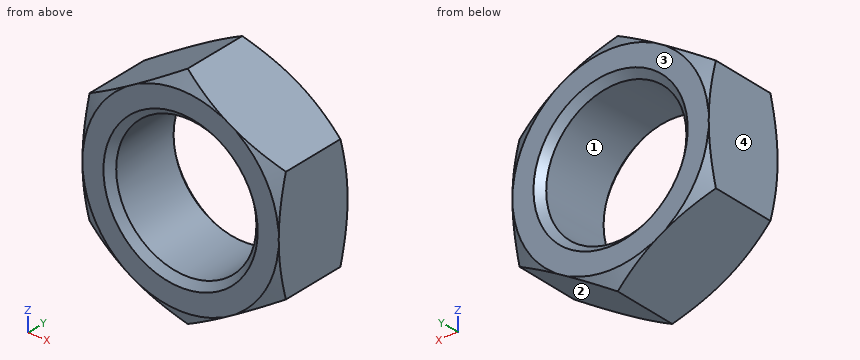
```python
from build123d import *

# Parameters (mm, degrees)
BOSS_EXTRUDE1_DEPTH = 6
SKETCH2_OUTSIDE_W   = 80.454
SKETCH2_OUTSIDE_H   = 84.786
SKETCH2_OUTSIDE_R   = 14
CUT_EXTRUDE1_DEPTH  = 12
CUT_EXTRUDE1_TAPER  = 60
SKETCH3_R           = 10
CUT_EXTRUDE2_DEPTH  = 13
CHAMFER1_SIZE       = 1


with BuildPart() as part:
    # Sketch1 → Boss-Extrude1 (new body, symmetric)
    with BuildSketch(Plane(origin=(0, 0, 0), x_dir=(1, 0, 0), z_dir=(0, 1, 0))):
        Polygon((14, 8.082903769), (0, 16.165807537), (-14, 8.082903769), (-14, -8.082903769), (0, -16.165807537), (14, -8.082903769), align=None)
    extrude(amount=BOSS_EXTRUDE1_DEPTH, both=True)

    # Sketch2 outside → Cut-Extrude1 (cut)
    with BuildSketch(Plane(origin=(0, 6, 0), x_dir=(1, 0, 0), z_dir=(0, 1, 0))):
        Rectangle(SKETCH2_OUTSIDE_W, SKETCH2_OUTSIDE_H)
        Circle(SKETCH2_OUTSIDE_R, mode=Mode.SUBTRACT)
    cut_extrude1 = extrude(amount=-CUT_EXTRUDE1_DEPTH, taper=CUT_EXTRUDE1_TAPER, mode=Mode.SUBTRACT)

    # Mirror1: Cut-Extrude1 across plane
    add(cut_extrude1.mirror(Plane.ZX), mode=Mode.SUBTRACT)

    # Sketch3 → Cut-Extrude2 (cut, through all)
    with BuildSketch(Plane(origin=(0, 6, 0), x_dir=(1, 0, 0), z_dir=(0, 1, 0))):
        Circle(SKETCH3_R)
    extrude(amount=-CUT_EXTRUDE2_DEPTH, mode=Mode.SUBTRACT)

    # Chamfer1
    chamfer1_edges = [part.edges().sort_by_distance(p)[0] for p in [
        (-10, -6, 0),
        (-10, 6, 0),
    ]]
    chamfer(chamfer1_edges, length=CHAMFER1_SIZE)


solid = part.part
```
The listing builds one solid part. Answer for the finished solid, in the listing's coordinates (mm). Face numbers are marked on the shaded views. Give positions to 0.01 mm unless a question says otherwise; leave off trailing zeros. Order: outer loops, then holes, each group sorted by start corner. A loop starts at its lowest first (then second) coordinate and runs counter-clockwise, first axis right, second up. Notation, with made-up numbers: (-23.75, -29.75) -> (34.25, -29.75) arc R28 cw to (34.25, 1.25) -> close; hole circle Ø11 at (13.25, 23.5). An arc over 180 degrees is marked (long way). Answer as CSV lines item,"result". Start each with the question number.
Q1. A cutting plane is placed at A-A (y = 3). Determine the outline of the cut face in (x, z), then the cut area to 3 significant figures.
Q2. Find the intervals of material crossed by L1, parallel to Z at x = 0, y = -1.75; L2, parallel to X at y = -1.75, z = 0; L3, parallel to Z at x = 8.5, y = -2, in increasing order.
Q3. Determine the mould class of the marked faces 1, 2, 3 and 4 for opening direction X: pulls with the +X half, pulls with the -X half, needs draft (parallel to the pull), parting line crosses it, or undercut.
Q4. Given pin 1 (5 mm diameter, centred on y = 3, z = 12, fed in from -X); pin 2 (1.5 mm diameter, centred on x = 10, z = 12, fed in from +Y); pin 3 (5 mm diameter, centred on x = 9.5, y = -2.5, fed in from -Z); pin 4 (6 mm diameter, centred on x = 8, y = -3.5, fed in from -Z), each flat-ended and moving along its own axis, determine where each tip first touches the part or whether it passes through.
Results found:
1,outline,"(-14, -8.08) -> (0, -16.17) -> (14, -8.08) -> (14, 8.08) -> (0, 16.17) -> (-14, 8.08) -> close; hole circle Ø20 at (0, 0)"
1,area,"365 mm2"
2,L1,"-16.17 to -10, 10 to 16.17"
2,L2,"-14 to -10, 10 to 14"
2,L3,"-11.26 to -5.27, 5.27 to 11.26"
3,face 1,"undercut"
3,face 2,"pulls with the +X half"
3,face 3,"needs draft"
3,face 4,"pulls with the -X half"
4,pin 1,"x = -11.55"
4,pin 2,"through"
4,pin 3,"z = -12.12"
4,pin 4,"z = -13.28"
